Source: CAD feature listing. Evaluate the final solid. Frame: model axes, mm. Coordinates: 2 decimals unless noted, no trailing zeros. Order: outer loops, then holes, each group sorted by start corner. A loop starts at its lowest first (then second) coordinate and runs counter-clockwise, first axis right, second up. Notation, with made-up numbers: (38, 38.5) - (71, 38.5) arc R16 cw to (71, 66.5) - close; hole circle Ø5 at (78, 69.25). An arc over 180 degrees is marked (long way). One line per question, with ' | ' between items. Start each with the question number.
(1) Contact query for a flat-ended pin moving along its axis: P1, Ø8, axis at x = 25.2, y = -55, coming from the -Z side. Output: stop coordinate, or through.
(2) Section C-C (z = 2.9). Count the separate pieces of the cut face and the enclosed holes in it, then the cut area to 3 significant figures.
(3) Section D-D (y = -60). Return the cut outline in (x, z), then the cut area to 3 significant figures.
(4) Section A-A (y = -30). Return the cut outline in (x, z).
(5) Section B-B (x = 25.2). Return the cut outline in (y, z).
(6) Line query: line 1 along Y through (x, z) = (0, 1.05); line 2 along X through (y, z) = (60, 0.8); line 3 along Y through (x, z) = (-24.8, 2.4). Output: solid intervals per line, ascending.
(7) Draft query along Y for faces 1 (the flat face through (-8, 1, 0)), 2 (the cylindrical face through (-0.099, -57.752, 0.764)), 3 (the cylindrical face through (22.7, -4.9, 2)), 4 (the flat face through (0, 75, 2)). Return one class per face: +Y half, -Y half, draft (parallel to the pull), parting line (faces both ways), or undercut.
Autodesk Inventor part; units mm, degrees
ref_plane "YZ Plane" through (0, 0, 0) normal (1, 0, 0) x (0, 1, 0)
ref_plane "XZ Plane" through (0, 0, 0) normal (0, 1, 0) x (-1, 0, 0)
ref_plane "XY Plane" through (0, 0, 0) normal (0, 0, 1) x (1, 0, 0)
sketch "Esboço1" plane through (0, 0, 0) normal (0, 0, 1) x (1, 0, 0)
  line L0 (-35, -75) -> (35, -75)
  line L1 (35, -75) -> (35, 75)
  line L2 (35, 75) -> (-35, 75)
  line L3 (-35, 75) -> (-35, -75)
  line L4 (-35, -75) -> (35, 75) construction
  line L5 (35, -75) -> (-35, 75) construction
  point P0 (0, 0)
  dimension "d0" = 150
  dimension "d1" = 70
extrude "Extrusão1" add sketch "Esboço1" along normal blind 4
sketch "Esboço2" plane through (0, 0, 4) normal (0, 0, 1) x (1, 0, 0)
  line L0 (35, 75) -> (-35, 75)
  line L1 (-35, -75) -> (35, -75)
  line L2 (-35, 75) -> (-35, -75)
  point P0 (0, 0)
  point P1 (0, 60)
  point P2 (0, -60)
  point P3 (0, 0)
  dimension "d4" = 15
  dimension "d5" = 15
  dimension "d6" = 35
  dimension "d7" = 35
hole "Furo1" at (0, 60, 4) at (0, -60, 4) at (0, 0, 4) direction (0, 0, -1) diameter 4.5 end through all countersink diameter 9.4 countersink angle 90
chamfer "Chanfro1" distance 2 angle 45 4 edges at (35, -75, 2) (-35, -75, 2) (35, 75, 2) (-35, 75, 2)
sketch "Esboço3" plane through (0, 0, 4) normal (0, 0, 1) x (1, 0, 0)
  circle A0 centre (-24.8, -5) radius 3.8 construction
  circle A1 centre (-24.8, -55) radius 3.8 construction
  circle A2 centre (25.2, -5) radius 3.8 construction
  circle A3 centre (25.2, -55) radius 3.8 construction
  circle A4 centre (-24.8, -55) radius 2.5
  circle A5 centre (25.2, -55) radius 2.5
  circle A6 centre (25.2, -5) radius 2.5
  circle A7 centre (-24.8, -5) radius 2.5
  point P0 (0, 0)
  dimension "d18" = 5
  dimension "d19" = 0
extrude "Extrusão2" cut sketch "Esboço3" against normal blind 10
sketch "Esboço4" plane through (0, 0, 4) normal (0, 0, 1) x (1, 0, 0)
  circle A0 centre (0.2, -30) radius 5.5
  circle A1 centre (0.2, -30) radius 7.5
  point P0 (0, 0)
  dimension "d24" = 15
extrude "Extrusão3" cut sketch "Esboço4" against normal through all contours A0 | A1
properties part number "Espaçador Bastidor" material "Poliacetal"
Response values:
1) P1: stops at z = 0
2) separate pieces: 1 | enclosed holes: 8 | area: 10,100 mm²
3) outline: (-35, 0) - (-2.25, 0) - (-2.25, 1.55) - (-4.7, 4) - (-35, 4) - close; (2.25, 0) - (35, 0) - (35, 4) - (4.7, 4) - (2.25, 1.55) - close | area: 256 mm²
4) outline: (-35, 0) - (-7.3, 0) - (-7.3, 4) - (-35, 4) - close; (7.7, 0) - (35, 0) - (35, 4) - (7.7, 4) - close
5) outline: (-75, 0) - (-57.5, 0) - (-57.5, 4) - (-75, 4) - close; (-52.5, 0) - (-7.5, 0) - (-7.5, 4) - (-52.5, 4) - close; (-2.5, 0) - (75, 0) - (75, 4) - (-2.5, 4) - close
6) line 1: y = -75 to -62.25, -57.75 to -37.5, -22.5 to -2.25, 2.25 to 57.75, 62.25 to 75 | line 2: x = -35 to -2.25, 2.25 to 35 | line 3: y = -75 to -57.5, -52.5 to -7.5, -2.5 to 75
7) face 1: draft | face 2: undercut | face 3: undercut | face 4: +Y half
